CAD build for the part. Positions are in the model's coordinates, mm. Face numbers are marked on the shaded views. A direction names the side the tool comes from. Round coordinates to 2 decimals unless told otherwise and drop trailing zeros. Order: outer loops, then holes, each group sorted by start corner. A loop starts at its lowest first (then second) coordinate and runs counter-clockwise, first axis right, second up.
```python
from build123d import *

# Parameters (mm, degrees)
F0_W     = 18
F0_H     = 8
F0_R     = 16.5
F0_W_2   = 8
F0_H_2   = 18
F1_DEPTH = 1
F2_DEPTH = 20
F4_DEPTH = 20
F6_DEPTH = 20


with BuildPart() as f1:
    # F0 (on Top) → F1 (new body)
    with BuildSketch(Plane.XY):
        with BuildLine():
            Line((45.2809703886, 40.8809703886), (-35.8809703886, 40.8809703886))
            ThreePointArc((-35.8809703886, 40.8809703886), (-39.4165042945, 39.4165042945), (-40.8809703886, 35.8809703886))
            Line((-40.8809703886, 35.8809703886), (-40.8809703886, -45.2809703886))
            ThreePointArc((-40.8809703886, -45.2809703886), (-39.4165042945, -48.8165042945), (-35.8809703886, -50.2809703886))
            Line((-35.8809703886, -50.2809703886), (45.2809703886, -50.2809703886))
            ThreePointArc((45.2809703886, -50.2809703886), (48.8165042945, -48.8165042945), (50.2809703886, -45.2809703886))
            Line((50.2809703886, -45.2809703886), (50.2809703886, 35.8809703886))
            ThreePointArc((50.2809703886, 35.8809703886), (48.8165042945, 39.4165042945), (45.2809703886, 40.8809703886))
        make_face()
        with Locations((-27.3089791051, -44.8809703886)):
            Rectangle(F0_W, F0_H, mode=Mode.SUBTRACT)
        with Locations((-7.9089791051, -44.8809703886)):
            Rectangle(F0_W, F0_H, mode=Mode.SUBTRACT)
        with Locations((-22.9809703886, -22.9809703886)):
            Circle(F0_R, mode=Mode.SUBTRACT)
        with Locations((11.4910208949, -44.8809703886)):
            Rectangle(F0_W, F0_H, mode=Mode.SUBTRACT)
        with Locations((30.8910208949, -44.8809703886)):
            Rectangle(F0_W, F0_H, mode=Mode.SUBTRACT)
        with Locations((44.8809703886, -30.8910208949)):
            Rectangle(F0_W_2, F0_H_2, mode=Mode.SUBTRACT)
        with Locations((22.9809703886, -22.9809703886)):
            Circle(F0_R, mode=Mode.SUBTRACT)
        with Locations((44.8809703886, -11.4910208949)):
            Rectangle(F0_W_2, F0_H_2, mode=Mode.SUBTRACT)
        with Locations((-22.9809703886, 22.9809703886)):
            Circle(F0_R, mode=Mode.SUBTRACT)
        with Locations((44.8809703886, 7.9089791051)):
            Rectangle(F0_W_2, F0_H_2, mode=Mode.SUBTRACT)
        with Locations((22.9809703886, 22.9809703886)):
            Circle(F0_R, mode=Mode.SUBTRACT)
        with Locations((44.8809703886, 27.3089791051)):
            Rectangle(F0_W_2, F0_H_2, mode=Mode.SUBTRACT)
        with Locations((-22.9809703886, 22.9809703886)):
            Circle(F0_R)
        with Locations((22.9809703886, 22.9809703886)):
            Circle(F0_R)
        with Locations((22.9809703886, -22.9809703886)):
            Circle(F0_R)
        with Locations((-22.9809703886, -22.9809703886)):
            Circle(F0_R)
        with Locations((44.8809703886, 27.3089791051)):
            Rectangle(F0_W_2, F0_H_2)
        with Locations((44.8809703886, 7.9089791051)):
            Rectangle(F0_W_2, F0_H_2)
        with Locations((44.8809703886, -11.4910208949)):
            Rectangle(F0_W_2, F0_H_2)
        with Locations((44.8809703886, -30.8910208949)):
            Rectangle(F0_W_2, F0_H_2)
        with Locations((30.8910208949, -44.8809703886)):
            Rectangle(F0_W, F0_H)
        with Locations((11.4910208949, -44.8809703886)):
            Rectangle(F0_W, F0_H)
        with Locations((-7.9089791051, -44.8809703886)):
            Rectangle(F0_W, F0_H)
        with Locations((-27.3089791051, -44.8809703886)):
            Rectangle(F0_W, F0_H)
    extrude(amount=-F1_DEPTH)

    # F0 (on Top) → F2 (join)
    with BuildSketch(Plane.XY):
        with BuildLine():
            Line((45.2809703886, 40.8809703886), (-35.8809703886, 40.8809703886))
            ThreePointArc((-35.8809703886, 40.8809703886), (-39.4165042945, 39.4165042945), (-40.8809703886, 35.8809703886))
            Line((-40.8809703886, 35.8809703886), (-40.8809703886, -45.2809703886))
            ThreePointArc((-40.8809703886, -45.2809703886), (-39.4165042945, -48.8165042945), (-35.8809703886, -50.2809703886))
            Line((-35.8809703886, -50.2809703886), (45.2809703886, -50.2809703886))
            ThreePointArc((45.2809703886, -50.2809703886), (48.8165042945, -48.8165042945), (50.2809703886, -45.2809703886))
            Line((50.2809703886, -45.2809703886), (50.2809703886, 35.8809703886))
            ThreePointArc((50.2809703886, 35.8809703886), (48.8165042945, 39.4165042945), (45.2809703886, 40.8809703886))
        make_face()
        with Locations((-27.3089791051, -44.8809703886)):
            Rectangle(F0_W, F0_H, mode=Mode.SUBTRACT)
        with Locations((-7.9089791051, -44.8809703886)):
            Rectangle(F0_W, F0_H, mode=Mode.SUBTRACT)
        with Locations((-22.9809703886, -22.9809703886)):
            Circle(F0_R, mode=Mode.SUBTRACT)
        with Locations((11.4910208949, -44.8809703886)):
            Rectangle(F0_W, F0_H, mode=Mode.SUBTRACT)
        with Locations((30.8910208949, -44.8809703886)):
            Rectangle(F0_W, F0_H, mode=Mode.SUBTRACT)
        with Locations((44.8809703886, -30.8910208949)):
            Rectangle(F0_W_2, F0_H_2, mode=Mode.SUBTRACT)
        with Locations((22.9809703886, -22.9809703886)):
            Circle(F0_R, mode=Mode.SUBTRACT)
        with Locations((44.8809703886, -11.4910208949)):
            Rectangle(F0_W_2, F0_H_2, mode=Mode.SUBTRACT)
        with Locations((-22.9809703886, 22.9809703886)):
            Circle(F0_R, mode=Mode.SUBTRACT)
        with Locations((44.8809703886, 7.9089791051)):
            Rectangle(F0_W_2, F0_H_2, mode=Mode.SUBTRACT)
        with Locations((22.9809703886, 22.9809703886)):
            Circle(F0_R, mode=Mode.SUBTRACT)
        with Locations((44.8809703886, 27.3089791051)):
            Rectangle(F0_W_2, F0_H_2, mode=Mode.SUBTRACT)
    extrude(amount=F2_DEPTH)

    # F3 (on face) → F4 (cut, through all)
    with BuildSketch(Plane.XY.offset(20)):
        with BuildLine():
            Line((22.9809703886, 39.4809703886), (-22.9809703886, 39.4809703886))
            ThreePointArc((-22.9809703886, 39.4809703886), (-11.313708499, 34.6482322781), (-6.4809703886, 22.9809703886))
            ThreePointArc((-6.4809703886, 22.9809703886), (-22.9809703886, 6.4809703886), (-39.4809703886, 22.9809703886))
            Line((-39.4809703886, 22.9809703886), (-39.4809703886, -22.9809703886))
            ThreePointArc((-39.4809703886, -22.9809703886), (-22.9809703886, -6.4809703886), (-6.4809703886, -22.9809703886))
            ThreePointArc((-6.4809703886, -22.9809703886), (-11.313708499, -34.6482322781), (-22.9809703886, -39.4809703886))
            Line((-22.9809703886, -39.4809703886), (22.9809703886, -39.4809703886))
            ThreePointArc((22.9809703886, -39.4809703886), (11.313708499, -11.313708499), (39.4809703886, -22.9809703886))
            Line((39.4809703886, -22.9809703886), (39.4809703886, 22.9809703886))
            ThreePointArc((39.4809703886, 22.9809703886), (11.313708499, 11.313708499), (22.9809703886, 39.4809703886))
        make_face()
    extrude(amount=-F4_DEPTH, mode=Mode.SUBTRACT)

    # F5 (on face) → F6 (join)
    with BuildSketch(Plane.XY.offset(20)):
        with BuildLine():
            ThreePointArc((50.2809703886, 35.8809703886), (48.8165042945, 39.4165042945), (45.2809703886, 40.8809703886))
            Line((45.2809703886, 40.8809703886), (-35.8809703886, 40.8809703886))
            ThreePointArc((-35.8809703886, 40.8809703886), (-39.4165042945, 39.4165042945), (-40.8809703886, 35.8809703886))
            Line((-40.8809703886, 35.8809703886), (-40.8809703886, -45.2809703886))
            ThreePointArc((-40.8809703886, -45.2809703886), (-39.4165042945, -48.8165042945), (-35.8809703886, -50.2809703886))
            Line((-35.8809703886, -50.2809703886), (45.2809703886, -50.2809703886))
            ThreePointArc((45.2809703886, -50.2809703886), (48.8165042945, -48.8165042945), (50.2809703886, -45.2809703886))
            Line((50.2809703886, -45.2809703886), (50.2809703886, 35.8809703886))
        make_face()
        with BuildLine():
            ThreePointArc((-39.4809703886, 35.8809703886), (-38.4265548008, 38.4265548008), (-35.8809703886, 39.4809703886))
            Line((-35.8809703886, 39.4809703886), (-22.9809703886, 39.4809703886))
            Line((-22.9809703886, 39.4809703886), (22.9809703886, 39.4809703886))
            Line((22.9809703886, 39.4809703886), (45.2809703886, 39.4809703886))
            ThreePointArc((45.2809703886, 39.4809703886), (47.6704440357, 38.5736299827), (48.8554365779, 36.3089791051))
            Line((48.8554365779, 36.3089791051), (48.8809703886, 36.3089791051))
            Line((48.8809703886, 36.3089791051), (48.8809703886, 35.8809703886))
            Line((48.8809703886, 35.8809703886), (48.8809703886, 18.3089791051))
            Line((48.8809703886, 18.3089791051), (48.8809703886, 16.9089791051))
            Line((48.8809703886, 16.9089791051), (48.8809703886, -1.0910208949))
            Line((48.8809703886, -1.0910208949), (48.8809703886, -2.4910208949))
            Line((48.8809703886, -2.4910208949), (48.8809703886, -20.4910208949))
            Line((48.8809703886, -20.4910208949), (48.8809703886, -21.8910208949))
            Line((48.8809703886, -21.8910208949), (48.8809703886, -39.8910208949))
            Line((48.8809703886, -39.8910208949), (48.8809703886, -45.2809703886))
            ThreePointArc((48.8809703886, -45.2809703886), (47.8265548008, -47.8265548008), (45.2809703886, -48.8809703886))
            Line((45.2809703886, -48.8809703886), (39.8910208949, -48.8809703886))
            Line((39.8910208949, -48.8809703886), (21.8910208949, -48.8809703886))
            Line((21.8910208949, -48.8809703886), (20.4910208949, -48.8809703886))
            Line((20.4910208949, -48.8809703886), (2.4910208949, -48.8809703886))
            Line((2.4910208949, -48.8809703886), (1.0910208949, -48.8809703886))
            Line((1.0910208949, -48.8809703886), (-16.9089791051, -48.8809703886))
            Line((-16.9089791051, -48.8809703886), (-18.3089791051, -48.8809703886))
            Line((-18.3089791051, -48.8809703886), (-35.8809703886, -48.8809703886))
            Line((-35.8809703886, -48.8809703886), (-36.3089791051, -48.8809703886))
            Line((-36.3089791051, -48.8809703886), (-36.3089791051, -48.8554365779))
            ThreePointArc((-36.3089791051, -48.8554365779), (-38.5736299827, -47.6704440357), (-39.4809703886, -45.2809703886))
            Line((-39.4809703886, -45.2809703886), (-39.4809703886, -22.9809703886))
            Line((-39.4809703886, -22.9809703886), (-39.4809703886, 22.9809703886))
            Line((-39.4809703886, 22.9809703886), (-39.4809703886, 35.8809703886))
        make_face(mode=Mode.SUBTRACT)
    extrude(amount=F6_DEPTH)


solid = f1.part
```
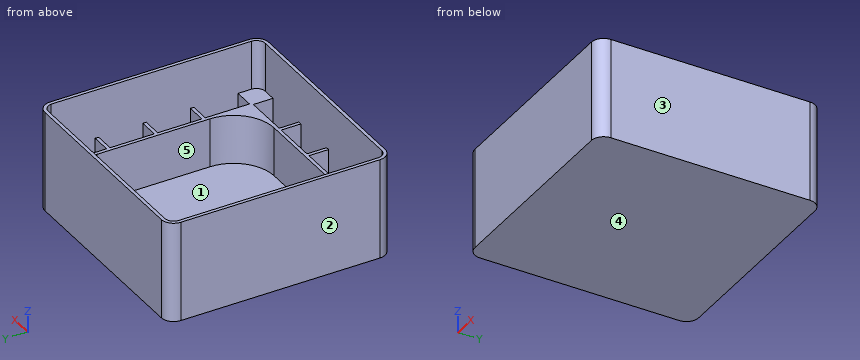
1. Tool access for the marked faces 4 and 5: list every direction of +Z, -Z, +X, -X, +Y, -Y with a clear straight run to the whole face (end or side of a thin tool).
2. Mould opens along X. For the marked faces 1, 2 and 3 say: released by +X, released by -X, zero draft, split by the parting line, or undercut.
3. Cut at A-A, the plane y = -6. Write the cut outline in (x, z).
4. Pin check, flat tip, straight feed: P1, Ø1.5, axis at x = 14.5, y = -27, coming from the +Z side. Stop position of the tip, or through.
5. Drill centre lines: line 1 (Y direction, x = -13, z = 12); line 2 (X direction, y = 12, z = 18); line 3 (Y direction, x = 10, z = 29). Where is each one in solid material? Low to high.
6. Cut at D-D, the plane z = 3. Give the number of separate pieces and of enclosed holes in the cut face, and give its area (3 significant figures).
7. Cut at C-C, the plane x = -14.5. Write the cut outline in (y, z).
Outcome:
1. face 4: -Z, +X, -X, +Y, -Y
1. face 5: +Z
2. face 1: undercut
2. face 2: released by -X
2. face 3: released by +X
3. outline: (-40.88, -1) - (50.28, -1) - (50.28, 40) - (48.88, 40) - (48.88, 0) - (40.88, 0) - (40.88, 20) - (39.48, 20) - (39.48, 0) - (-39.48, 0) - (-39.48, 40) - (-40.88, 40) - close
4. P1: stops at z = 0
5. line 1: y = -50.28 to -48.88, -40.88 to -39.48, 39.48 to 40.88
5. line 2: x = -40.88 to -39.48, 39.48 to 40.88, 48.88 to 50.28
5. line 3: y = -50.28 to -48.88, 39.48 to 40.88
6. separate pieces: 1
6. enclosed holes: 9
6. area: 1,140 mm2
7. outline: (-50.28, -1) - (40.88, -1) - (40.88, 40) - (39.48, 40) - (39.48, 0) - (-39.48, 0) - (-39.48, 20) - (-40.88, 20) - (-40.88, 0) - (-48.88, 0) - (-48.88, 40) - (-50.28, 40) - close
